Can you work these out from the drawing? Everything is in mm from the part's minimum corner. A direction names the side the tool comes from. Round coordinates to 2 decimals unless told otherwise and drop trailing zeros. Write each loop counter-clockwise with the first axis right and the second up, starting at its lowest first coordinate (ties: lowest second). Pieces come first, ordered by that corner, then holes. Notation, with made-up numbers: M 51,49 L 96,49 A10 cw 96,61 Z; hole C -17.75,-20 d9. An arc over 180 degrees is marked long. Use a Markdown table: item, result. Add a question column.
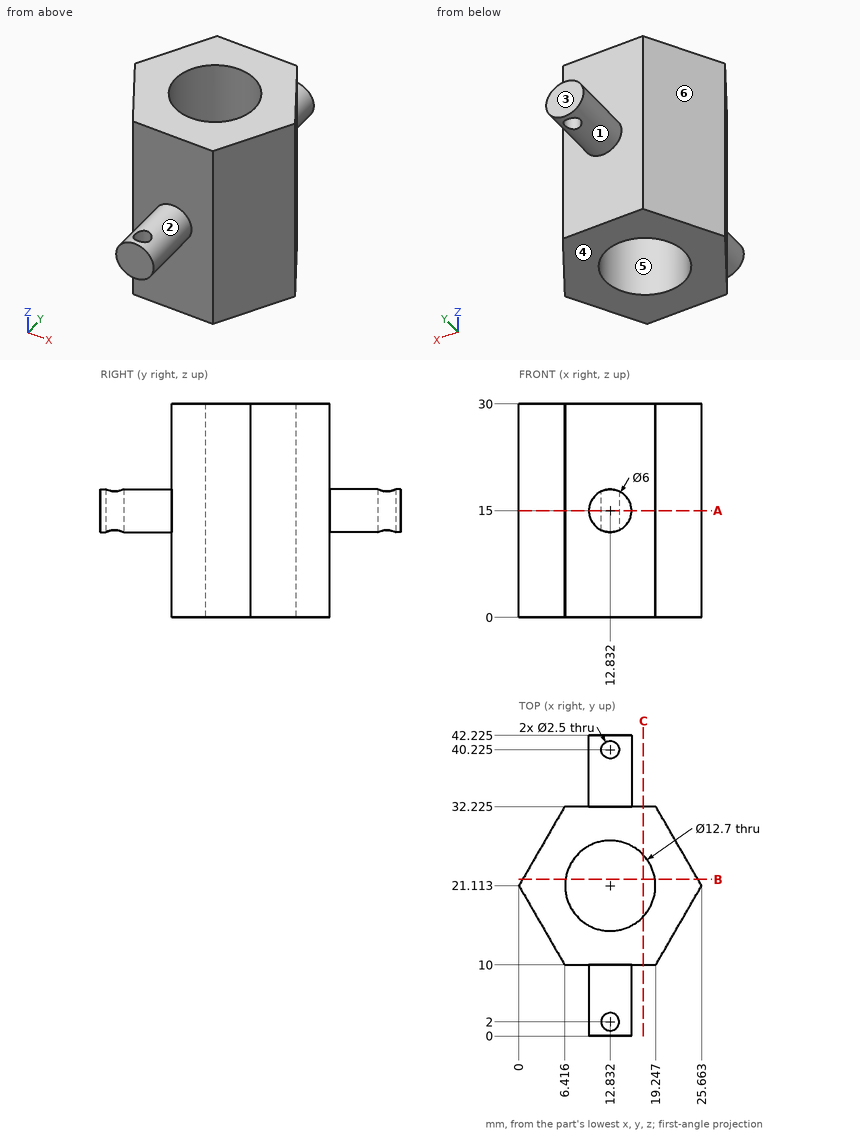
Item 1: I need wall thicknesses on probe 1 along X at (y, z) = (24.5, 28) (1 decimal); probe 2 along X at (y, z) = (40.5, 15); probe 3 along Y at (x, z) = (22, 24.5) (1 decimal). Which ranges of each line are inside material? Lowest first, please. Write a range as from..to.
Item 2: If we mould it in two halves opening along X, with no side actions, what happens to the marked faces 4, 5 and 6? For each: +X half, -X half, draft (parallel to the pull), parting line (faces both ways), or undercut.
Item 3: Imagine slicing it at A-A on z = 15. Count the separate pieces of the cut face and the enclosed holes in it, plus the area to 3 significant figures.
Item 4: For pin 1 Ø1.5 at (x, z) = (6.5, 6.5) entering from +Y (1 decimal); pin 2 Ø2 at (x, z) = (5.5, 10.5) entering from -Y; pin 3 Ø4 at (x, y) = (12.83, 40.23) entering from +Z, each with a flat end and sliding along its axis, tell me the tip position at first contact or that it passes through.
Item 5: On a 3-axis mill with a long thin cutter (end or side, diameter ignored), from which of +Z, -Z, +X, -X, +Y, -Y can I reach the whole of each face in a straight line? I mean the marked faces 1, 2 and 3. Say none if no direction works.
Item 6: Imagine slicing it at B-B on y = 22. List the corners of the cut face in (x, z) for me, plus the area to 3 significant figures.
Item 7: Imagine slicing it at C-C on x = 17.5. List the corners of the cut face in (y, z) for me (1 decimal).
The answers:
| question | item | result |
|---|---|---|
| 1 | probe 1 | 2..7.5, 18.2..23.7 |
| 1 | probe 2 | 9.83..11.61, 14.05..15.83 |
| 1 | probe 3 | 14.8..27.5 |
| 2 | face 4 | draft |
| 2 | face 5 | undercut |
| 2 | face 6 | -X half |
| 3 | separate pieces | 1 |
| 3 | enclosed holes | 3 |
| 3 | area | 411 mm² |
| 4 | pin 1 | y = 32.2 |
| 4 | pin 2 | y = 10 |
| 4 | pin 3 | z = 18 |
| 5 | face 1 | +Y |
| 5 | face 2 | -Y |
| 5 | face 3 | +Z, -Z, +X, -X, +Y |
| 6 | outline | M 0.51,0 L 6.54,0 L 6.54,30 L 0.51,30 Z; M 19.12,0 L 25.15,0 L 25.15,30 L 19.12,30 Z |
| 6 | area | 362 mm² |
| 7 | outline | M 10,0 L 16.8,0 L 16.8,30 L 10,30 Z; M 25.4,0 L 32.2,0 L 32.2,30 L 25.4,30 Z |
